Part model, mm, in its own coordinate system. A direction names the side the tool comes from. Round coordinates to 2 decimals unless told otherwise and drop trailing zeros. Order: outer loops, then holes, each group sorted by start corner. A loop starts at its lowest first (then second) coordinate and runs counter-clockwise, first axis right, second up. Notation, with made-up numbers: (18.25, 43.25) -> (39.25, 43.25) arc R20 ccw to (39.25, 58.25) -> close; hole circle Ø11 at (71.25, 40.5). An arc over 180 degrees is marked (long way). Answer as a JSON object with one key per item and string values. Group by question number.
Autodesk Inventor part; units mm, degrees
ref_plane "YZ Plane" through (0, 0, 0) normal (1, 0, 0) x (0, 1, 0)
ref_plane "XZ Plane" through (0, 0, 0) normal (0, 1, 0) x (-1, 0, 0)
ref_plane "XY Plane" through (0, 0, 0) normal (0, 0, 1) x (1, 0, 0)
sketch "Sketch1" plane through (0, 0, 0) normal (0, 0, 1) x (1, 0, 0)
  line L0 (0, 0) -> (50, 0) construction
  line L1 (0, 0) -> (37.5, 0)
  line L2 (37.5, 0) -> (34.5, 0)
  line L3 (34.5, 0) -> (34.5, 5)
  line L4 (34.5, 5) -> (53, 5)
  line L5 (53, 5) -> (53, -5)
  line L6 (53, -5) -> (34.5, -5)
  line L7 (34.5, -5) -> (34.5, 5)
  line L8 (0, 0) -> (37.1652, 5) construction
  line L9 (0, 0) -> (37.1652, -5) construction
  arc A0 (37.1652, -5) -> (37.1652, 5) centre (0, 0) ccw
  line L10 (0, 0) -> (49.7494, 5) construction
  arc A1 (49.7494, -5) -> (49.7494, 5) centre (0, 0) ccw
  line L11 (34.5, -5) -> (53, -5)
  line L12 (53, -5) -> (53, -3)
  line L13 (53, -3) -> (34.5, -3)
  line L14 (34.5, -3) -> (34.5, -5)
  line L15 (34.5, 5) -> (53, 5)
  line L16 (53, 5) -> (53, 3)
  line L17 (53, 3) -> (34.5, 3)
  line L18 (34.5, 3) -> (34.5, 5)
  line L19 (37.1652, -5) -> (36.1652, -5)
  arc A2 (36.1652, -5) -> (36.1652, 5) centre (-1, 0) ccw
  line L20 (49.7494, -5) -> (50.7494, -5)
  arc A3 (50.7494, -5) -> (50.7494, 5) centre (1, 0) ccw
  point P0 (36.3798, 3)
  point P1 (36.3798, -3)
  point P2 (50.9099, -3)
  point P3 (50.9099, 3)
  dimension "d7" = 50
  dimension "d8" = 37.5
  dimension "d9" = 3
  dimension "d10" = 5
  dimension "d11" = 18.5
  dimension "d12" = 10
  dimension "d13" = 37.5
  dimension "d14" = 50
  dimension "d15" = 2
  dimension "d16" = 2
  dimension "d17" = 1
  dimension "d18" = 1
extrude "Extrusion1" add sketch "Sketch1" along normal blind 1
extrude "Extrusion2" add sketch "Sketch1" along normal blind 3 contours L3 L4 A2 L17 | L13 A2 L6 L7 | L13 A0 L6 A2 | A2 L4 A0 L17 | L13 A1 L6 A0 | A0 L4 A1 L17 | L13 A3 L6 A1 | A1 L4 A3 L17 | L13 L5 L6 A3 | A3 L4 L5 L17
extrude "Extrusion3" add sketch "Sketch1" against normal blind 20 contours A2 L17 A0 L1 | L1 A0 L13 A2 | L3 L4 A2 L17 | L13 A2 L6 L7 | L13 A0 L6 A2 | A2 L4 A0 L17 | L13 A3 L6 A1 | A1 L17 A3 L13 | A1 L4 A3 L17 | L13 L5 L6 A3 | A3 L4 L5 L17
properties part number "Coils" material "Stainless Steel"
Q1. Which spindle directions (+Z, -Z, +X, -X, +Y, -Y) get a long thin tool onto all of the face, cutting with end or side? Do faces 1 (the cylindrical face through (51, 0, -10)), 2 (the cylindrical face through (36.5, 0, -9.9)), 3 (the flat face through (44, 0, 1)), 4 (the flat face through (50, -5, -6)). Say none if no direction does.
Q2. Two-plate mould, pull along X, no slides. Class faces 5 (the flat face through (52, 0, 0)), 6 (the cylindrical face through (50, 0, -10)), 7 (the cylindrical face through (37.5, -0.1, -9.9)), 8 (the flat face through (34.5, -3.4, -8.7)): +X half, -X half, draft (parallel to the pull), parting line (faces both ways), or undercut.
Q3. Band-saw the part on B-B (x = 41). List the corners of the cut face in (y, z).
Q4. Drop flat-ended pins along their axis: pin 1 Ø1.5 at (x, y) = (42.5, 1.5) entering from -Z; pin 2 Ø6 at (y, z) = (1, -3) entering from -X; pin 3 Ø10 at (x, z) = (43, -17.5) entering from -Y. Give the stop position or say it passes through.
Q5. Band-saw the part on A-A (z = -11.25). List the corners of the cut face in (x, y).
Q6. Wall check: line 1 (Y direction, x = 36, z = -16); line 2 (Z direction, x = 37, y = -0.75); line 3 (Z direction, x = 35.75, y = -1.5). Give the ranges that are in metal, low to high. Write a range as [from, to].
Q7. Band-saw the part on D-D (x = 36.75). List the corners of the cut face in (y, z), plus the area to 3 significant figures.
Q8. Band-saw the part on C-C (y = 2.75). List the corners of the cut face in (x, z).
Completed:
{
 "1": {"face 1": "-Z, +X", "face 2": "-Z, -X", "face 3": "+Z, +X, -X", "face 4": "+Z, -Z, +X, -X, -Y"},
 "2": {"face 5": "draft", "face 6": "undercut", "face 7": "undercut", "face 8": "-X half"},
 "3": {"outline": "(-5, 0) -> (5, 0) -> (5, 3) -> (3, 3) -> (3, 1) -> (-3, 1) -> (-3, 3) -> (-5, 3) -> close"},
 "4": {"pin 1": "z = 0", "pin 2": "x = 34.5", "pin 3": "through"},
 "5": {"outline": "(34.5, -5) -> (37.17, -5) arc R37.5 ccw to (37.17, 5) -> (34.5, 5) -> (34.5, 3) -> (36.38, 3) arc R37.5 cw to (36.38, -3) -> (34.5, -3) -> close; (49.75, -5) -> (53, -5) -> (53, -3) -> (50.91, -3) arc R50 ccw to (50.91, 3) -> (53, 3) -> (53, 5) -> (49.75, 5) arc R50 cw to start"},
 "6": {"line 1": "[-5, -3], [3, 5]", "line 2": "[-20, 1]", "line 3": "[0, 1]"},
 "7": {"outline": "(-5, -20) -> (5, -20) -> (5, 3) -> (3, 3) -> (3, 1) -> (-3, 1) -> (-3, 3) -> (-5, 3) -> close", "area": "218 mm2"},
 "8": {"outline": "(34.5, 0) -> (36.4, 0) -> (36.4, -20) -> (37.4, -20) -> (37.4, 0) -> (49.92, 0) -> (49.92, -20) -> (50.92, -20) -> (50.92, 0) -> (53, 0) -> (53, 1) -> (34.5, 1) -> close"}
}
